Design review of the part built by this model. Coordinates are the model's own, in mm. A direction names the side the tool comes from. Round coordinates to 2 decimals unless told otherwise and drop trailing zeros. Write each loop counter-clockwise with the first axis right and the second up, starting at its lowest first coordinate (ties: lowest second). Pieces come first, ordered by that corner, then holes. Notation, with made-up numbers: (3.25, -17.5) -> (20.25, -17.5) arc R18 cw to (20.25, -1.5) -> close; hole circle Ø1 at (3.25, 31). An arc over 180 degrees is marked (long way). Write item = value, one per line. Start each with the question number.
Item 1: For pin 1 Ø2.5 at (y, z) = (-1, 32.5) entering from -X; pin 2 Ø1 at (x, y) = (3.5, 3) entering from -Z; pin 3 Ø3 at (x, z) = (13.5, 40.5) entering from -Y, all flat-tipped, find the tip position at first contact; note any pin that passes through.
Item 2: Add section D-D, the plane x = 8.25. State the section outline as (y, z) points, then the cut area to 3 significant figures.
Item 3: Add section B-B, the plane z = 47. State the section outline as (x, y) points, then the cut area to 3 significant figures.
Item 4: Mouldability with a two-part tool opening along X and no side actions: class faces 1 (the flat face through (3, 0, 19.05)), 2 (the flat face through (13, 0, 35.56)), 3 (the flat face through (12.02, 0, 44)) as released by +X, released by -X, zero draft, split by the parting line, or undercut.
Item 5: Add section A-A, the plane z = 33. State the section outline as (x, y) points.
Item 6: To check wall thickness, follow L1, parallel to X at y = 0, z = 14.25; L2, parallel to Z at x = -3.75, y = 0.5; L3, parallel to Z at x = -1.75, y = 9. State the ranges of each line that lie inside material, in increasing order.
Item 7: Machinability: for faces 4 (the flat face through (10.75, 0, 32)), 5 (the flat face through (0, -7, 38.1)), 6 (the flat face through (-2, 9, 35.56)), 7 (the flat face through (13, 2.297, 41)), 8 (the flat face through (13, -2.297, 41)), which of the approach directions +Z, -Z, +X, -X, +Y, -Y give a long, thin tool a straight path to every point of the face, cutting with its end or side? Answer none if there is none.
Item 8: Add section C-C, the plane z = 8. State the section outline as (x, y) points (1 decimal).
from build123d import *

# Parameters (mm, degrees)
F0_R     = 8.5725
F1_DEPTH = 25.4
F3_DEPTH = 12.7
F4_R     = 7.261951
F5_DEPTH = 19.05
F6_DEPTH = 25.4
F7_DEPTH = 10.16


with BuildPart() as f1:
    # F0 (on Top) → F1 (new body)
    with BuildSketch(Plane.XY):
        with Locations((3.447682, 0)):
            Circle(F0_R)
    extrude(amount=F1_DEPTH)

    # F2 (on face) → F3 (join)
    with BuildSketch(Plane.XY.offset(25.4)):
        with BuildLine():
            Line((-2.192824, -5.175653), (-2.671089, -6.004032))
            ThreePointArc((-2.671089, -6.004032), (-1.803051, -6.77625), (-0.838568, -7.424003))
            ThreePointArc((-0.838568, -7.424003), (0.204643, -7.935393), (1.307422, -8.301027))
            Line((1.307422, -8.301027), (1.785687, -7.472648))
            Line((1.785687, -7.472648), (-2.192824, -5.175653))
        make_face()
        with BuildLine():
            ThreePointArc((1.307422, 8.301027), (0.204643, 7.935393), (-0.838568, 7.424003))
            ThreePointArc((-0.838568, 7.424003), (-1.803396, 6.775982), (-2.671701, 6.003408))
            Line((-2.671701, 6.003408), (-2.195779, 5.173949))
            Line((-2.195779, 5.173949), (1.785687, 7.472648))
            Line((1.785687, 7.472648), (1.307422, 8.301027))
        make_face()
        with BuildLine():
            ThreePointArc((12.020182, 0), (11.941453, 1.159143), (11.706711, 2.296994))
            Line((11.706711, 2.296994), (10.750182, 2.296994))
            Line((10.750182, 2.296994), (10.750182, -2.296994))
            Line((10.750182, -2.296994), (11.706711, -2.296994))
            ThreePointArc((11.706711, -2.296994), (11.941453, -1.159143), (12.020182, 0))
        make_face()
        with BuildLine():
            Line((12.020182, 0), (12.020182, 2.296994))
            Line((12.020182, 2.296994), (11.706711, 2.296994))
            ThreePointArc((11.706711, 2.296994), (11.941453, 1.159143), (12.020182, 0))
        make_face()
        with BuildLine():
            Line((12.020182, -2.296994), (12.020182, 0))
            ThreePointArc((12.020182, 0), (11.941453, -1.159143), (11.706711, -2.296994))
            Line((11.706711, -2.296994), (12.020182, -2.296994))
        make_face()
        with BuildLine():
            Line((-2.671089, -6.004032), (-2.827824, -6.275506))
            Line((-2.827824, -6.275506), (-0.838568, -7.424003))
            ThreePointArc((-0.838568, -7.424003), (-1.803051, -6.77625), (-2.671089, -6.004032))
        make_face()
        with BuildLine():
            ThreePointArc((1.307422, -8.301027), (0.204643, -7.935393), (-0.838568, -7.424003))
            Line((-0.838568, -7.424003), (1.150687, -8.5725))
            Line((1.150687, -8.5725), (1.307422, -8.301027))
        make_face()
        with BuildLine():
            Line((1.150687, 8.5725), (-0.838568, 7.424003))
            ThreePointArc((-0.838568, 7.424003), (0.204643, 7.935393), (1.307422, 8.301027))
            Line((1.307422, 8.301027), (1.150687, 8.5725))
        make_face()
        with BuildLine():
            Line((-0.838568, 7.424003), (-2.827824, 6.275506))
            Line((-2.827824, 6.275506), (-2.671701, 6.003408))
            ThreePointArc((-2.671701, 6.003408), (-1.803396, 6.775982), (-0.838568, 7.424003))
        make_face()
    extrude(amount=F3_DEPTH)

    # F4 (on face) → F5 (cut)
    with BuildSketch(Plane(origin=(0, 0, 0), x_dir=(1, 0, 0), z_dir=(0, 0, -1))):
        with Locations((3.447682, 0)):
            Circle(F4_R)
    extrude(amount=-F5_DEPTH, mode=Mode.SUBTRACT)

    # F2 (on face) → F6 (join)
    with BuildSketch(Plane.XY.offset(25.4)):
        Polygon((-0.838568, -7.424003), (-2.827824, -6.275506), (-4.097824, -8.47521), (-0.119313, -10.772205), (1.150687, -8.5725), align=None)
        Polygon((14.560182, 2.296994), (12.020182, 2.296994), (12.020182, 0), (12.020182, -2.296994), (14.560182, -2.296994), align=None)
        Polygon((-4.097824, 8.47521), (-2.827824, 6.275506), (-0.838568, 7.424003), (1.150687, 8.5725), (-0.119313, 10.772205), align=None)
    extrude(amount=F6_DEPTH)

    # F2 (on face) → F7 (cut)
    with BuildSketch(Plane.XY.offset(25.4)):
        Polygon((-0.838568, -7.424003), (-2.827824, -6.275506), (-4.097824, -8.47521), (-0.119313, -10.772205), (1.150687, -8.5725), align=None)
        Polygon((14.560182, 2.296994), (12.020182, 2.296994), (12.020182, 0), (12.020182, -2.296994), (14.560182, -2.296994), align=None)
        Polygon((-4.097824, 8.47521), (-2.827824, 6.275506), (-0.838568, 7.424003), (1.150687, 8.5725), (-0.119313, 10.772205), align=None)
    extrude(amount=F7_DEPTH, mode=Mode.SUBTRACT)


solid = f1.part
Result set:
q1.pin_1 = 10.75
q1.pin_2 = 19.05
q1.pin_3 = -2.3
q2.outline = (-7.1, 0) -> (-5.45, 0) -> (-5.45, 19.05) -> (5.45, 19.05) -> (5.45, 0) -> (7.1, 0) -> (7.1, 25.4) -> (-7.1, 25.4) -> close
q2.area = 153 mm²
q3.outline = (-4.1, -8.48) -> (-0.12, -10.77) -> (1.15, -8.57) -> (-0.84, -7.42) -> (-2.83, -6.28) -> close; (-4.1, 8.48) -> (-2.83, 6.28) -> (-0.84, 7.42) -> (1.15, 8.57) -> (-0.12, 10.77) -> close; (12.02, -2.3) -> (14.56, -2.3) -> (14.56, 2.3) -> (12.02, 2.3) -> close
q3.area = 35.0 mm²
q4.face_1 = undercut
q4.face_2 = zero draft
q4.face_3 = released by -X
q5.outline = (-2.83, -6.28) -> (-0.84, -7.42) -> (1.15, -8.57) -> (1.31, -8.3) -> (1.79, -7.47) -> (-2.19, -5.18) -> (-2.67, -6) -> close; (-2.83, 6.28) -> (-2.67, 6) -> (-2.2, 5.17) -> (1.79, 7.47) -> (1.31, 8.3) -> (1.15, 8.57) -> (-0.84, 7.42) -> close; (10.75, -2.3) -> (12.02, -2.3) -> (12.02, 2.3) -> (10.75, 2.3) -> close
q6.L1 = -5.12 to -3.81, 10.71 to 12.02
q6.L2 = 19.05 to 25.4
q6.L3 = 35.56 to 50.8
q7.face_4 = +Z, -X, +Y, -Y
q7.face_5 = +Z, +X
q7.face_6 = -Z, -X, +Y
q7.face_7 = +Z, +X, -X, +Y
q7.face_8 = +Z, +X, -X, -Y
q8.outline = circle Ø17.1 at (3.4, 0); hole circle Ø14.5 at (3.4, 0)
